Here's how the part is built. I have some questions about the finished solid (model axes, mm). A direction names the side the tool comes from. Round coordinates to 2 decimals unless told otherwise and drop trailing zeros. Order: outer loops, then holes, each group sorted by start corner. A loop starts at its lowest first (then second) coordinate and runs counter-clockwise, first axis right, second up. Notation, with made-up numbers: (27, 47.5) -> (44, 47.5) arc R34 cw to (44, 83.5) -> close; hole circle Ø5 at (38.5, -24). An arc over 180 degrees is marked (long way). One line per item, written item: value.
```python
from build123d import *

# Parameters (mm, degrees)
BOSS_EXTRUDE1_DEPTH = 8.89
SKETCH2_R           = 2.54
CUT_EXTRUDE1_DEPTH  = 28.94
SKETCH3_R           = 2.54
CUT_EXTRUDE2_DEPTH  = 28.94
SKETCH4_R           = 2.54
CUT_EXTRUDE3_DEPTH  = 8.89


with BuildPart() as part:
    # Sketch1 → Boss-Extrude1 (new body)
    with BuildSketch(Plane(origin=(0, 0, 0), x_dir=(1, 0, 0), z_dir=(0, 1, 0))):
        Polygon((6.35, 0), (-6.35, 0), (-25.68448, -25.4), (-34.57448, -25.4), (-34.57448, -27.94), (-25.68448, -27.94), (-6.35, -2.54), (6.35, -2.54), (25.68448, -27.94), (34.57448, -27.94), (34.57448, -25.4), (25.68448, -25.4), align=None)
    extrude(amount=BOSS_EXTRUDE1_DEPTH)

    # Sketch2 → Cut-Extrude1 (cut, through all)
    with BuildSketch(Plane.XY.offset(27.94)):
        with Locations((-30.12948, 4.445)):
            Circle(SKETCH2_R)
    extrude(amount=-CUT_EXTRUDE1_DEPTH, mode=Mode.SUBTRACT)

    # Sketch3 → Cut-Extrude2 (cut, through all)
    with BuildSketch(Plane.XY.offset(27.94)):
        with Locations((30.12948, 4.445)):
            Circle(SKETCH3_R)
    extrude(amount=-CUT_EXTRUDE2_DEPTH, mode=Mode.SUBTRACT)

    # Sketch4 → Cut-Extrude3 (cut)
    with BuildSketch(Plane.XY.offset(2.54)):
        with Locations((0, 4.445)):
            Circle(SKETCH4_R)
    extrude(amount=-CUT_EXTRUDE3_DEPTH, mode=Mode.SUBTRACT)


solid = part.part
```
Q1. For P1, Ø1, axis at x = 8.5, y = 3, coming from the +Z side; P2, Ø4.5, axis at x = 0.5, y = 4.5, coming from the +Z side; P3, Ø3, axis at x = 10.5, y = 2.5, coming from the +Z side, each with a flat end and sliding along its axis, tell me the tip position at first contact or that it passes through.
Answers:
P1: z = 6.02
P2: z = 2.54
P3: z = 9.96
Q2. I need wall thicknesses on line 1 along Y through (x, z) = (0, 1.75) (3 decimals); line 2 along Z through (x, y) = (-2, 7.5); line 3 along X through (y, z) = (4, 5.25). Which ranges of each line are inside material? Lowest first, please.
Answers:
line 1: 0 to 1.905, 6.985 to 8.89
line 2: 0 to 2.54
line 3: -10.35 to -8.41, 8.41 to 10.35
Q3. I want a section at D-D on z = 26.25. Write out the boundary of the cut face in (x, y) (3 decimals).
Answers:
outline: (-34.574, 0) -> (-24.398, 0) -> (-24.398, 8.89) -> (-34.574, 8.89) -> close; (24.398, 0) -> (34.574, 0) -> (34.574, 8.89) -> (24.398, 8.89) -> close; hole circle Ø5.08 at (-30.129, 4.445); hole circle Ø5.08 at (30.129, 4.445)
Q4. Which directions (+Z, -Z, +X, -X, +Y, -Y) give clear straight access to the entire face, cutting with the end or side of a thin tool? Please do faces 1 (the face through (10, 0, 7)), 2 (the face through (-3, 4, 0)), 3 (the face through (32, 2, 25.4)), 4 (the face through (-32, 2, 25.4)), 5 (the face through (-16.153, 4.383, 15.418)).
Answers:
face 1: +Z, -Z, +X, -X, -Y
face 2: -Z, +X, -X, +Y, -Y
face 3: -Z, +X, +Y, -Y
face 4: -Z, -X, +Y, -Y
face 5: +Z, +Y, -Y
Q5. I want a section at A-A on x = 0. Write out the boundary of the cut face in (y, z) (3 decimals), then the cut area to 3 significant figures.
Answers:
outline: (0, 0) -> (1.905, 0) -> (1.905, 2.54) -> (0, 2.54) -> close; (6.985, 0) -> (8.89, 0) -> (8.89, 2.54) -> (6.985, 2.54) -> close
area: 9.68 mm2
Q6. I want a section at C-C on z = 8.75. Write out the boundary of the cut face in (x, y).
Answers:
outline: (-13.01, 0) -> (-11.08, 0) -> (-11.08, 8.89) -> (-13.01, 8.89) -> close; (11.08, 0) -> (13.01, 0) -> (13.01, 8.89) -> (11.08, 8.89) -> close
Q7. I want a section at B-B on y = 8.25. Write out the boundary of the cut face in (x, z), then the cut area to 3 significant figures.
Answers:
outline: (-34.57, 25.4) -> (-25.68, 25.4) -> (-6.35, 0) -> (6.35, 0) -> (25.68, 25.4) -> (34.57, 25.4) -> (34.57, 27.94) -> (25.68, 27.94) -> (6.35, 2.54) -> (-6.35, 2.54) -> (-25.68, 27.94) -> (-34.57, 27.94) -> close
area: 176 mm2
